Input: part model. Units: mm. Frame: model coordinates. Round coordinates to 2 decimals unless told otherwise and drop trailing zeros. Order: outer loops, then holes, each group sorted by start corner. A loop starts at its lowest first (then second) coordinate and runs counter-clockwise, first axis right, second up.
Item 1: Cut plane A-A on y = 283. Output: boundary loops of the cut face in (x, z) (3 decimals), then the cut area to 3 significant figures.
Item 2: First-contact query: pin 1 (4 mm diameter, centred on x = 118, y = 606.5, fed in from +Z); pin 2 (4 mm diameter, centred on x = 323.5, y = 207, fed in from +Z) (3 decimals). Flat tips, straight axial feed; report the tip coordinate or a pass-through.
Item 3: Line query: L1, parallel to X at y = 418, z = -8.5. Output: solid intervals per line, ascending.
Item 4: Cut plane B-B on z = -3. Give the number of separate pieces and of enclosed holes in the cut face, then the cut area to 3 significant figures.
```python
from build123d import *

# Parameters (mm, degrees)
SKETCH002_W           = 20.05
SKETCH002_H           = 1270
EXTRUDE002_DEPTH      = 12.7
EXTRUDE002_DEPTH_BACK = 10.525
SKETCH001_R           = 3.96875
EXTRUDE001_DEPTH      = 19.05
EXTRUDE001_DEPTH_BACK = 16.05
EXTRUDE_DEPTH         = 1219.2
BOX_W                 = 980
BOX_H                 = 900
BOX_DEPTH             = 50


with BuildPart() as extrude002:
    # Sketch002 (on Face1 of Cut) → Extrude002 (new body, two sides)
    with BuildSketch(Plane.XY) as extrude002_sk:
        with Locations((187.825, -609.6)):
            Rectangle(SKETCH002_W, SKETCH002_H)
        with Locations((467.225, -609.6)):
            Rectangle(SKETCH002_W, SKETCH002_H)
        with Locations((746.625, -609.6)):
            Rectangle(SKETCH002_W, SKETCH002_H)
        with Locations((1026.025, -609.6)):
            Rectangle(SKETCH002_W, SKETCH002_H)
    extrude(amount=EXTRUDE002_DEPTH)
    extrude(extrude002_sk.sketch, amount=-EXTRUDE002_DEPTH_BACK)


with BuildPart() as extrude001:
    # Sketch001 (on Face1 of Extrude) → Extrude001 (new body, two sides)
    with BuildSketch(Plane.XY) as extrude001_sk:
        with Locations((254, -152.4)):
            Circle(SKETCH001_R)
        with Locations((330.2, -152.4)):
            Circle(SKETCH001_R)
        with Locations((406.4, -152.4)):
            Circle(SKETCH001_R)
        with Locations((254, -228.6)):
            Circle(SKETCH001_R)
        with Locations((406.4, -228.6)):
            Circle(SKETCH001_R)
        with Locations((254, -304.8)):
            Circle(SKETCH001_R)
        with Locations((330.2, -304.8)):
            Circle(SKETCH001_R)
        with Locations((406.4, -304.8)):
            Circle(SKETCH001_R)
        with Locations((253.99999, -381)):
            Circle(SKETCH001_R)
        with Locations((330.19999, -381)):
            Circle(SKETCH001_R)
        with Locations((406.39999, -381)):
            Circle(SKETCH001_R)
        with Locations((253.99999, -457.2)):
            Circle(SKETCH001_R)
        with Locations((406.39999, -457.2)):
            Circle(SKETCH001_R)
        with Locations((253.99999, -533.4)):
            Circle(SKETCH001_R)
        with Locations((330.19999, -533.4)):
            Circle(SKETCH001_R)
        with Locations((406.39999, -533.4)):
            Circle(SKETCH001_R)
        with Locations((253.99998, -609.6)):
            Circle(SKETCH001_R)
        with Locations((330.19998, -609.6)):
            Circle(SKETCH001_R)
        with Locations((406.39998, -609.6)):
            Circle(SKETCH001_R)
        with Locations((253.99998, -685.8)):
            Circle(SKETCH001_R)
        with Locations((406.39998, -685.8)):
            Circle(SKETCH001_R)
        with Locations((253.99998, -762)):
            Circle(SKETCH001_R)
        with Locations((330.19998, -762)):
            Circle(SKETCH001_R)
        with Locations((406.39998, -762)):
            Circle(SKETCH001_R)
        with Locations((253.99997, -838.2)):
            Circle(SKETCH001_R)
        with Locations((330.19997, -838.2)):
            Circle(SKETCH001_R)
        with Locations((406.39997, -838.2)):
            Circle(SKETCH001_R)
        with Locations((253.99997, -914.4)):
            Circle(SKETCH001_R)
        with Locations((406.39997, -914.4)):
            Circle(SKETCH001_R)
        with Locations((253.99997, -990.6)):
            Circle(SKETCH001_R)
        with Locations((330.19997, -990.6)):
            Circle(SKETCH001_R)
        with Locations((406.39997, -990.6)):
            Circle(SKETCH001_R)
        with Locations((533.4, -152.4)):
            Circle(SKETCH001_R)
        with Locations((609.6, -152.4)):
            Circle(SKETCH001_R)
        with Locations((685.8, -152.4)):
            Circle(SKETCH001_R)
        with Locations((533.4, -228.6)):
            Circle(SKETCH001_R)
        with Locations((685.8, -228.6)):
            Circle(SKETCH001_R)
        with Locations((533.4, -304.8)):
            Circle(SKETCH001_R)
        with Locations((609.6, -304.8)):
            Circle(SKETCH001_R)
        with Locations((685.8, -304.8)):
            Circle(SKETCH001_R)
        with Locations((533.39999, -381)):
            Circle(SKETCH001_R)
        with Locations((609.59999, -381)):
            Circle(SKETCH001_R)
        with Locations((685.79999, -381)):
            Circle(SKETCH001_R)
        with Locations((533.39999, -457.2)):
            Circle(SKETCH001_R)
        with Locations((685.79999, -457.2)):
            Circle(SKETCH001_R)
        with Locations((533.39999, -533.4)):
            Circle(SKETCH001_R)
        with Locations((609.59999, -533.4)):
            Circle(SKETCH001_R)
        with Locations((685.79999, -533.4)):
            Circle(SKETCH001_R)
        with Locations((533.39998, -609.6)):
            Circle(SKETCH001_R)
        with Locations((609.59998, -609.6)):
            Circle(SKETCH001_R)
        with Locations((685.79998, -609.6)):
            Circle(SKETCH001_R)
        with Locations((533.39998, -685.8)):
            Circle(SKETCH001_R)
        with Locations((685.79998, -685.8)):
            Circle(SKETCH001_R)
        with Locations((533.39998, -762)):
            Circle(SKETCH001_R)
        with Locations((609.59998, -762)):
            Circle(SKETCH001_R)
        with Locations((685.79998, -762)):
            Circle(SKETCH001_R)
        with Locations((533.39997, -838.2)):
            Circle(SKETCH001_R)
        with Locations((609.59997, -838.2)):
            Circle(SKETCH001_R)
        with Locations((685.79997, -838.2)):
            Circle(SKETCH001_R)
        with Locations((533.39997, -914.4)):
            Circle(SKETCH001_R)
        with Locations((685.79997, -914.4)):
            Circle(SKETCH001_R)
        with Locations((533.39997, -990.6)):
            Circle(SKETCH001_R)
        with Locations((609.59997, -990.6)):
            Circle(SKETCH001_R)
        with Locations((685.79997, -990.6)):
            Circle(SKETCH001_R)
        with Locations((812.8, -152.4)):
            Circle(SKETCH001_R)
        with Locations((889, -152.4)):
            Circle(SKETCH001_R)
        with Locations((965.2, -152.4)):
            Circle(SKETCH001_R)
        with Locations((812.8, -228.6)):
            Circle(SKETCH001_R)
        with Locations((965.2, -228.6)):
            Circle(SKETCH001_R)
        with Locations((812.8, -304.8)):
            Circle(SKETCH001_R)
        with Locations((889, -304.8)):
            Circle(SKETCH001_R)
        with Locations((965.2, -304.8)):
            Circle(SKETCH001_R)
        with Locations((812.79999, -381)):
            Circle(SKETCH001_R)
        with Locations((888.99999, -381)):
            Circle(SKETCH001_R)
        with Locations((965.19999, -381)):
            Circle(SKETCH001_R)
        with Locations((812.79999, -457.2)):
            Circle(SKETCH001_R)
        with Locations((965.19999, -457.2)):
            Circle(SKETCH001_R)
        with Locations((812.79999, -533.4)):
            Circle(SKETCH001_R)
        with Locations((888.99999, -533.4)):
            Circle(SKETCH001_R)
        with Locations((965.19999, -533.4)):
            Circle(SKETCH001_R)
        with Locations((812.79998, -609.6)):
            Circle(SKETCH001_R)
        with Locations((888.99998, -609.6)):
            Circle(SKETCH001_R)
        with Locations((965.19998, -609.6)):
            Circle(SKETCH001_R)
        with Locations((812.79998, -685.8)):
            Circle(SKETCH001_R)
        with Locations((965.19998, -685.8)):
            Circle(SKETCH001_R)
        with Locations((812.79998, -762)):
            Circle(SKETCH001_R)
        with Locations((888.99998, -762)):
            Circle(SKETCH001_R)
        with Locations((965.19998, -762)):
            Circle(SKETCH001_R)
        with Locations((812.79997, -838.2)):
            Circle(SKETCH001_R)
        with Locations((888.99997, -838.2)):
            Circle(SKETCH001_R)
        with Locations((965.19997, -838.2)):
            Circle(SKETCH001_R)
        with Locations((812.79997, -914.4)):
            Circle(SKETCH001_R)
        with Locations((965.19997, -914.4)):
            Circle(SKETCH001_R)
        with Locations((812.79997, -990.6)):
            Circle(SKETCH001_R)
        with Locations((888.99997, -990.6)):
            Circle(SKETCH001_R)
        with Locations((965.19997, -990.6)):
            Circle(SKETCH001_R)
    extrude(amount=EXTRUDE001_DEPTH)
    extrude(extrude001_sk.sketch, amount=-EXTRUDE001_DEPTH_BACK)


with BuildPart() as cut001:
    # Sketch → Extrude (new body)
    with BuildSketch(Plane.XZ):
        Polygon((0, 0), (1219.2, 0), (1219.2, -12.7), (1193.8, -12.7), (1193.8, -19.05), (25.4, -19.05), (25.4, -12.7), (0, -12.7), align=None)
    extrude(amount=EXTRUDE_DEPTH)

    # Cut: cut Extrude001
    add(extrude001.part, mode=Mode.SUBTRACT)

    # Cut001: cut Extrude002
    add(extrude002.part, mode=Mode.SUBTRACT)


with BuildPart() as cut001_1:
    # Cut001 placement: moved
    add(cut001.part.moved(Location((-136.2, 1140.396, 0))))


with BuildPart() as common:
    # Box → Box (new body)
    with BuildSketch(Plane.XY.offset(-49)):
        with Locations((490, 450)):
            Rectangle(BOX_W, BOX_H)
    extrude(amount=BOX_DEPTH)

    # Common: intersect Cut001
    add(cut001_1.part, mode=Mode.INTERSECT)


solid = common.part
```
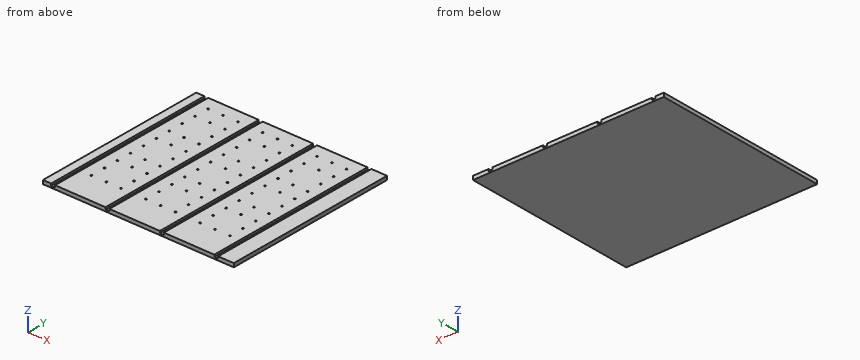
From the geometry:
1. outline: (0, -19.05) - (980, -19.05) - (980, 0) - (899.85, 0) - (899.85, -10.525) - (879.8, -10.525) - (879.8, 0) - (620.45, 0) - (620.45, -10.525) - (600.4, -10.525) - (600.4, 0) - (341.05, 0) - (341.05, -10.525) - (321, -10.525) - (321, 0) - (61.65, 0) - (61.65, -10.525) - (41.6, -10.525) - (41.6, 0) - (0, 0) - close
1. area: 17,800 mm2
2. pin 1: stops at z = -16.05
2. pin 2: stops at z = -10.525
3. L1: x = 0 to 41.6, 61.65 to 321, 341.05 to 600.4, 620.45 to 879.8, 899.85 to 980
4. separate pieces: 5
4. enclosed holes: 81
4. area: 806,000 mm2
